The listing builds one solid part. Answer for the finished solid, in the listing's coordinates (mm). Face numbers are marked on the shaded views. A direction names the side the tool comes from. Round coordinates to 2 decimals unless told otherwise and drop trailing zeros. Loops run counter-clockwise (first coordinate to the right, second up) from the corner with the lowest first, then second, coordinate; pieces in that order, holes last. Notation, with made-up numbers: (88, -4.5) -> (112, -4.5) arc R27 cw to (112, 29.5) -> close; hole circle Ø9 at (-7.75, 0). An arc over 180 degrees is marked (long way). Use a Markdown table: item, result. Add a question column.
Q1. Section C-C on x = -2 is taken. Give the vertices of the cut face in (y, z), then the cut area to 3 significant figures.
Q2. Section B-B on z = 1 is taken. Give the vertices of the cut face in (x, y), then the cut area to 3 significant figures.
Q3. Consider line 1 (Z direction, x = 7.5, y = 2.5); line 2 (X direction, y = 2.75, z = 0.75); line 3 (Z direction, x = 9.5, y = -7). Determine where each line is inside the solid, lowest interval first.
Q4. Given pin 1 Ø1.1 at (x, z) = (25.5, 9.5) entering from +Y; pin 2 Ø10 at (x, y) = (17.5, -0.5) entering from +Z; pin 3 Ø4 at (y, z) = (5.5, 3.5) entering from +X, each flat-ended and moving along its own axis, determine where each tip first touches the part or whether it passes through.
Q5. Section D-D on y = -3.5 is taken. Give the vertices of the cut face in (x, z), then the cut area to 3 significant figures.
Q6. For a pull along Y with two mould halves and no side action, classify the marked faces 6, 7 and 8 as released by +Y, released by -Y, zero draft, split by the parting line, or undercut.
Q7. Which of the six approach directions +Z, -Z, +X, -X, +Y, -Y give full straight-line access (tool end or side, diameter ignored) to the marked faces 1, 2, 3, 4 and 5?
Q8. Section A-A on x = 5 is taken. Give the vertices of the cut face in (y, z).
from build123d import *

# Parameters (mm, degrees)
F0_W      = 20
F0_H      = 20
F0_W_2    = 12
F0_H_2    = 15.4
F1_DEPTH  = 2
F2_W      = 15.9
F2_H      = 20
F3_DEPTH  = 1
F4_W      = 2
F4_H      = 20
F5_DEPTH  = 7
F7_DEPTH  = 3.001
F9_DEPTH  = 2.3
F11_DEPTH = 4
F12_W     = 20
F12_H     = 2
F13_DEPTH = 16.8
F14_W     = 15
F14_H     = 2
F15_DEPTH = 2.7
F16_W     = 15
F16_H     = 2.88
F16_H_2   = 2
F17_DEPTH = 4.88
F19_DEPTH = 17.501
F20_W     = 15
F20_H     = 3.7
F21_DEPTH = 8.4
F23_DEPTH = 17.501
F24_W     = 1
F24_H     = 5
F25_DEPTH = 1.5
F26_R     = 1
F27_R     = 1


with BuildPart() as f1:
    # F0 (on Top) → F1 (new body)
    with BuildSketch(Plane.XY):
        Rectangle(F0_W, F0_H)
        Rectangle(F0_W_2, F0_H_2, mode=Mode.SUBTRACT)
    extrude(amount=F1_DEPTH)

    # F2 (on face) → F3 (join)
    with BuildSketch(Plane.XY.offset(2)):
        Rectangle(F2_W, F2_H)
    extrude(amount=F3_DEPTH)

    # F4 (on face) → F5 (join)
    with BuildSketch(Plane.XY.offset(3)):
        with Locations((-6.95, 0)):
            Rectangle(F4_W, F4_H)
    extrude(amount=F5_DEPTH)

    # F6 (on face) → F7 (cut, through all)
    with BuildSketch(Plane.XY.offset(3)):
        Polygon((0, 7.5), (-4.25, 7.5), (-4.25, -2.7), (-2.45, -2.7), (-2.45, 6.5), (0, 6.5), (2.45, 6.5), (2.45, -2.7), (4.25, -2.7), (4.25, 7.5), align=None)
    extrude(amount=-F7_DEPTH, mode=Mode.SUBTRACT)

    # F8 (on face) → F9 (join)
    with BuildSketch(Plane(origin=(0, 0, 2), x_dir=(1, 0, 0), z_dir=(0, 0, -1))):
        Polygon((1.5, -3.7), (0, -3.7), (-1.5, -3.7), (-1.5, -6.5), (1.5, -6.5), align=None)
    extrude(amount=F9_DEPTH)

    # F10 (on face) → F11 (cut)
    with BuildSketch(Plane.YZ.offset(1.5)):
        Polygon((5.847163, -0.3), (3.7, 2), (3.7, -0.3), align=None)
    extrude(amount=-F11_DEPTH, mode=Mode.SUBTRACT)

    # F12 (on face) → F13 (join)
    with BuildSketch(Plane.YZ.offset(-5.95)):
        with Locations((0, 9)):
            Rectangle(F12_W, F12_H)
    extrude(amount=F13_DEPTH)

    # F14 (on face) → F15 (join)
    with BuildSketch(Plane.YZ.offset(10.85)):
        with Locations((0, 9)):
            Rectangle(F14_W, F14_H)
    extrude(amount=F15_DEPTH)

    # F16 (on face) → F17 (join)
    with BuildSketch(Plane.YZ.offset(13.55)):
        with Locations((0, 6.56)):
            Rectangle(F16_W, F16_H)
        with Locations((0, 9)):
            Rectangle(F16_W, F16_H_2)
    extrude(amount=F17_DEPTH)

    # F18 (on face) → F19 (cut, through all)
    with BuildSketch(Plane.XZ.offset(7.5)):
        Polygon((18.43, 10), (13.55, 10), (18.43, 7.12), align=None)
        Polygon((18.43, 5.12), (13.55, 8), (13.55, 5.12), align=None)
    extrude(amount=-F19_DEPTH, mode=Mode.SUBTRACT)

    # F20 (on face) → F21 (join)
    with BuildSketch(Plane.YZ.offset(18.43)):
        with Locations((0, 6.97)):
            Rectangle(F20_W, F20_H)
    extrude(amount=F21_DEPTH)

    # F22 (on face) → F23 (cut, through all)
    with BuildSketch(Plane.XZ.offset(7.5)):
        Polygon((21.63, 7.12), (24.83, 8.82), (18.43, 8.82), (18.43, 7.12), align=None)
        Polygon((26.83, 5.12), (26.83, 8.256902), (21.63, 5.12), align=None)
    extrude(amount=-F23_DEPTH, mode=Mode.SUBTRACT)

    # F24 (on face) → F25 (join)
    with BuildSketch(Plane.XY.offset(8.82)):
        with Locations((25.83, 0)):
            Rectangle(F24_W, F24_H)
    extrude(amount=F25_DEPTH)

    # F26
    f26_edges = [f1.edges().sort_by_distance(p)[0] for p in [
        (25.83, -7.5, 8.82),
        (25.83, 7.5, 8.82),
        (26.83, -7.5, 8.538451),
        (26.83, 7.5, 8.538451),
    ]]
    fillet(f26_edges, radius=F26_R)

    # F27
    f27_edges = [f1.edges().sort_by_distance(p)[0] for p in [
        (10, -10, 1),
        (-10, -10, 1),
        (-10, 10, 1),
        (10, 10, 1),
        (10.85, 10, 9),
        (10.85, -10, 9),
    ]]
    fillet(f27_edges, radius=F27_R)


solid = f1.part
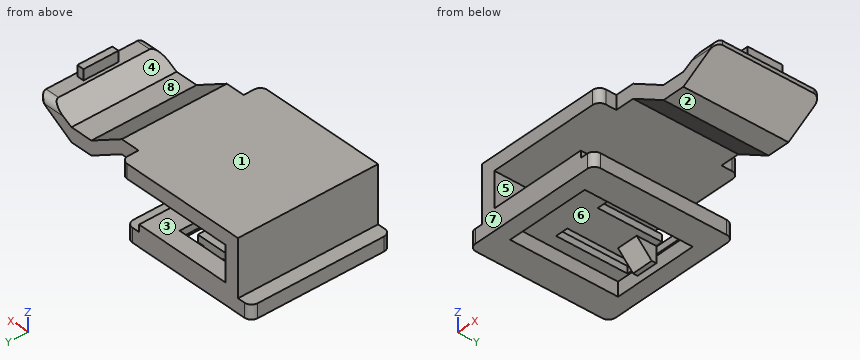
Checked values:
| question | item | result |
|---|---|---|
| 1 | outline | (-10, 0) -> (-7.7, 0) -> (-7.7, 2) -> (6.5, 2) -> (6.5, 3) -> (-10, 3) -> close; (-10, 8) -> (10, 8) -> (10, 10) -> (-10, 10) -> close; (7.5, 2) -> (7.7, 2) -> (7.7, 0) -> (10, 0) -> (10, 3) -> (7.5, 3) -> close |
| 1 | area | 68.2 mm2 |
| 2 | outline | (-10, -9) arc R1 ccw to (-9, -10) -> (9, -10) arc R1 ccw to (10, -9) -> (10, 9) arc R1 ccw to (9, 10) -> (-9, 10) arc R1 ccw to (-10, 9) -> close; (-1.5, 4.63) -> (1.5, 4.63) -> (1.5, 6.5) -> (-1.5, 6.5) -> close; hole (-6, -7.7) -> (6, -7.7) -> (6, 7.7) -> (-6, 7.7) -> close |
| 2 | area | 220 mm2 |
| 3 | line 1 | z = 0 to 3, 8 to 10 |
| 3 | line 2 | x = -10 to -6, 6 to 10 |
| 3 | line 3 | z = 0 to 2, 8 to 10 |
| 4 | pin 1 | stops at y = 2.5 |
| 4 | pin 2 | stops at z = 10 |
| 4 | pin 3 | stops at x = 22.26 |
| 5 | outline | (-10, 0) -> (-6, 0) -> (-6, 2) -> (6, 2) -> (6, 0) -> (10, 0) -> (10, 2) -> (7.95, 2) -> (7.95, 3) -> (-5.95, 3) -> (-5.95, 8) -> (13.55, 8) -> (18.43, 5.12) -> (21.63, 5.12) -> (26.83, 8.26) -> (26.83, 8.82) -> (24.83, 8.82) -> (21.63, 7.12) -> (18.43, 7.12) -> (13.55, 10) -> (-7.95, 10) -> (-7.95, 2) -> (-10, 2) -> close |
| 5 | area | 109 mm2 |
| 6 | face 6 | undercut |
| 6 | face 7 | released by -Y |
| 6 | face 8 | zero draft |
| 7 | face 1 | +Z, -X, +Y, -Y |
| 7 | face 2 | -Z, +X, +Y, -Y |
| 7 | face 3 | +X, +Y, -Y |
| 7 | face 4 | +Z, +Y, -Y |
| 7 | face 5 | +Y, -Y |
| 8 | outline | (-10, 0) -> (-7.7, 0) -> (-7.7, 2) -> (7.7, 2) -> (7.7, 0) -> (10, 0) -> (10, 3) -> (-10, 3) -> close; (-10, 8) -> (10, 8) -> (10, 10) -> (-10, 10) -> close |
